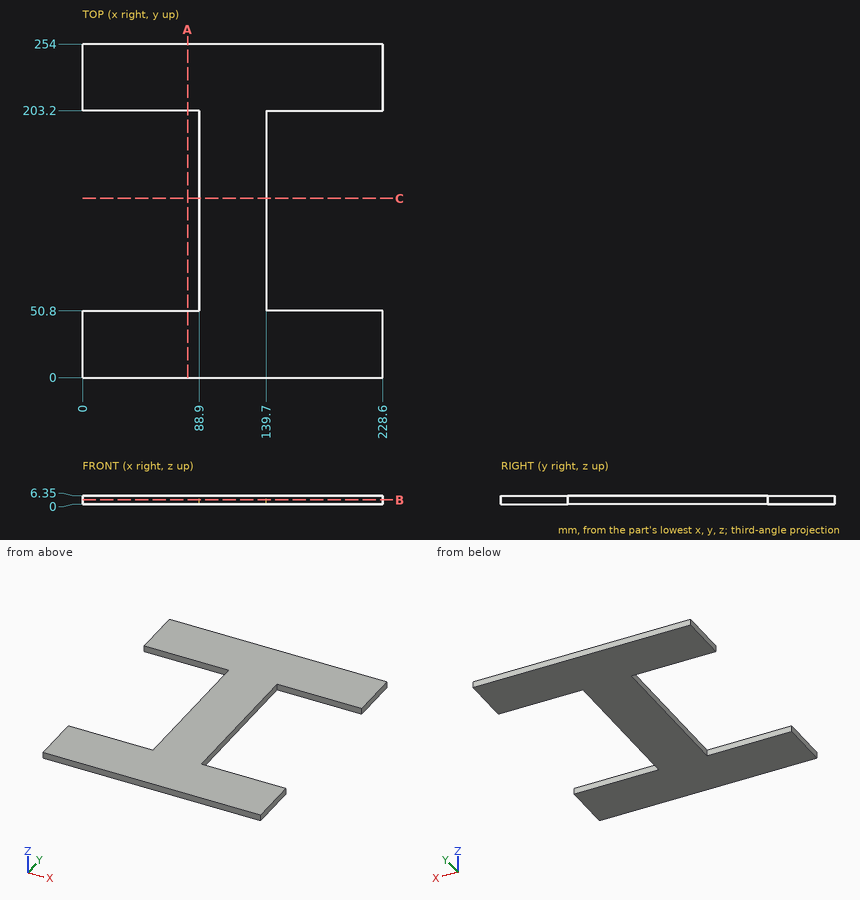
Drawing for the job (mm, zero at the part's lowest x, y, z). Coordinates: 2 decimals unless noted, no trailing zeros. Order: outer loops, then holes, each group sorted by start corner. A loop starts at its lowest first (then second) coordinate and runs counter-clockwise, first axis right, second up.
Item 1: Drill centre lines: L1, parallel to Y at x = 77.5, z = 2.75; L2, parallel to X at y = 179, z = 1.75. Where is each one in solid material? Low to high.
Check sheet entries:
L1: y = 0 to 50.8, 203.2 to 254
L2: x = 88.9 to 139.7
Item 2: Band-saw the part on A-A on x = 80. List the corners of the cut face in (y, z), plus the area to 3 significant figures.
Check sheet entries:
outline: (0, 0) - (50.8, 0) - (50.8, 6.35) - (0, 6.35) - close; (203.2, 0) - (254, 0) - (254, 6.35) - (203.2, 6.35) - close
area: 645 mm2
Item 3: Band-saw the part on C-C on y = 136.5. List the corners of the cut face in (x, z), plus the area to 3 significant figures.
Check sheet entries:
outline: (88.9, 0) - (139.7, 0) - (139.7, 6.35) - (88.9, 6.35) - close
area: 323 mm2
Item 4: Band-saw the part on B-B on z = 3.25. List the corners of the cut face in (x, y).
Check sheet entries:
outline: (0, 0) - (228.6, 0) - (228.6, 50.8) - (139.7, 50.8) - (139.7, 203.2) - (228.6, 203.2) - (228.6, 254) - (0, 254) - (0, 203.2) - (88.9, 203.2) - (88.9, 50.8) - (0, 50.8) - close
Item 5: Pin check, flat tips, straight feed: pin 1 Ø2 at (y, z) = (168.5, 5.5) entering from +X; pin 2 Ø1.9 at (y, z) = (104, 4) entering from -X. Stop position of each tip, or through.
Check sheet entries:
pin 1: stops at x = 139.7
pin 2: stops at x = 88.9
